from build123d import *

# Parameters (mm, degrees)
F2_DEPTH          = 3
F6_DEPTH          = 1.5
F9_DEPTH          = 26.2
F9_DEPTH_BACK     = 25
F10_R             = 1.5
F11_DEPTH         = 20
F13_R             = 2.25
F14_DEPTH         = 2
F14_COPIES2_COUNT = 2
F14_COPIES2_PITCH = 38.242646
F15_W             = 29
F15_H             = 11
F16_DEPTH         = 0.75


# Not quite as in the source:
# - a pattern or mirror of a feature is missing from the dataset's text; its kind, count and spacing are read off the source's solid


with BuildPart() as f2:
    # F1 (on offset) → F2 (new body)
    with BuildSketch(Plane.XY.offset(3.5)):
        Polygon((-11.75, -15.25), (-11.75, -2.5), (-11.75, 2.5), (-11.75, 15.25), (-16.75, 15.25), (-16.75, 0), (-16.75, -15.25), align=None)
        Polygon((0, -2.5), (11.75, -2.5), (11.75, 2.5), (0, 2.5), (-11.75, 2.5), (-11.75, -2.5), align=None)
        Polygon((16.75, -15.25), (16.75, 0), (16.75, 15.25), (11.75, 15.25), (11.75, 2.5), (11.75, -2.5), (11.75, -15.25), align=None)
    extrude(amount=F2_DEPTH)

    # F5 (on plane+point) → F6 (join, symmetric)
    with BuildSketch(Plane.YZ.offset(14.25)):
        Polygon((10.057664814, 6.5), (13.25, 6.5), (1.5, 38.8), (0, 38.8), (-1.5, 38.8), (-13.25, 6.5), (-10.057664814, 6.5), (-1.5, 30.0244743399), (0, 30.0244743399), (1.5, 30.0244743399), align=None)
    f6 = extrude(amount=F6_DEPTH, both=True)

    # F6_copies: F6 across plane
    add(f6.mirror(Plane(origin=(0, 0, 0), x_dir=(0, 0, -1), z_dir=(-1, 0, 0))))

    # F8 (on face) → F9 (join, two sides)
    with BuildSketch(Plane.XY.offset(38.8)) as f9_sk:
        with BuildLine():
            ThreePointArc((14.25, -1.5), (15.3106601718, -1.0606601718), (15.75, 0))
            ThreePointArc((15.75, 0), (15.3106601718, 1.0606601718), (14.25, 1.5))
            ThreePointArc((14.25, 1.5), (13.1893398223, 1.0606601659), (12.75, -1.67e-08))
            ThreePointArc((12.75, -1.67e-08), (13.1893398341, -1.0606601777), (14.25, -1.5))
        make_face()
    f9 = extrude(amount=F9_DEPTH) + extrude(f9_sk.sketch, amount=-F9_DEPTH_BACK)

    # F9_copies: F9 across plane
    add(f9.mirror(Plane(origin=(0, 0, 0), x_dir=(0, 0, -1), z_dir=(-1, 0, 0))))

    # F10 (on Right) → F11 (join, symmetric)
    with BuildSketch(Plane.YZ):
        with Locations((0, 65)):
            Circle(F10_R)
    extrude(amount=F11_DEPTH, both=True)

    # F13 (on offset) → F14 (join)
    with BuildSketch(Plane.XZ.offset(13.75)):
        with Locations((14.25, 2.25)):
            Circle(F13_R)
    f14 = extrude(amount=-F14_DEPTH)

    # F14_copies: F14 across plane
    add(f14.mirror(Plane.ZX))

    # F14_copies1: F14 across plane
    add(f14.mirror(Plane(origin=(0, 0, 0), x_dir=(0, 0, -1), z_dir=(-1, 0, 0))))

    # F14_copies2: F14 ×2
    with Locations(*[Vector(-0.7452413135, 0.6667948595, 0) * (i * F14_COPIES2_PITCH) for i in range(1, F14_COPIES2_COUNT)]):
        add(f14)

    # F15 (on Front) → F16 (join, symmetric)
    with BuildSketch(Plane.XZ):
        with Locations((0, 71.5)):
            Rectangle(F15_W, F15_H)
    extrude(amount=F16_DEPTH, both=True)


solid = f2.part
Design review of the part built by this model. Coordinates are the model's own, in mm. A direction names the side the tool comes from. Round coordinates to 2 decimals unless told otherwise and drop trailing zeros. Write each loop counter-clockwise with the first axis right and the second up, starting at its lowest first coordinate (ties: lowest second). Pieces come first, ordered by that corner, then holes.
Item 1: Consider section C-C on z = 59.5. Give the boundary of the cut face in (x, y).
Item 2: Consider section A-A on x = -1. Give the boundary of the cut face in (y, z).
Item 3: For faces 1 (the flat face through (11.75, 9, 5)), 2 (the flat face through (15.4, 1.2, 38.8)), 3 (the flat face through (-11.75, -9, 5)), list the 3-axis set-ups (+Z, -Z, +X, -X, +Y, -Y) from which the entire face can be reached by the end or side of a thin tool; tool diameter is ignored.
Item 4: Consider section B-B on z = 2.25. Give the boundary of the cut face in (x, y).
Item 5: Draft analysis for pull direction Z (two halves, no side actions). For faces 4 (the flat face through (14.27, 7.46, 22.42)), 5 (the flat face through (-14.5, 0, 72)), 6 (the flat face through (13.1, 1.2, 30.024)), state which applies: released by +Z, released by -Z, zero draft, split by the parting line, or undercut.
Item 6: For pin 1 Ø5 at (y, z) = (-10, 12.5) entering from -X; pin 2 Ø4 at (x, y) = (10, 6) entering from -Z; pin 3 Ø1.2 at (y, z) = (0, 70) entering from -X; pin 4 Ø4 at (x, z) = (8, 9) entering from +Y, all flat-tipped, find the tip position at first contact; note any pin that passes through.
Item 7: Wall thickness on L1, parallel to Z at x = 6, y = -2; L2, parallel to Y at x = 15, z = 15; L3, parallel to Y at x = 7, z = 72: over which ranges is each line inside the solid? List them lowest first.
Item 8: Consider section D-D on y = 5. Give the boundary of the cut face in (x, z).
Check values:
1. outline: circle Ø3 at (-14.25, 0); circle Ø3 at (14.25, 0)
2. outline: (-2.5, 3.5) - (2.5, 3.5) - (2.5, 6.5) - (-2.5, 6.5) - close; (-0.75, 66.3) arc R1.5 ccw (long way) to (0.75, 66.3) - (0.75, 77) - (-0.75, 77) - close
3. face 1: +Z, -Z, +Y
3. face 2: +X, +Y
3. face 3: +Z, -Z, -Y
4. outline: (-16.5, -13.75) - (-12, -13.75) - (-12, -11.75) - (-16.5, -11.75) - close; (-16.5, 11.75) - (-12, 11.75) - (-12, 13.75) - (-16.5, 13.75) - close; (12, -13.75) - (16.5, -13.75) - (16.5, -11.75) - (12, -11.75) - close; (12, 11.75) - (16.5, 11.75) - (16.5, 13.75) - (12, 13.75) - close
5. face 4: released by +Z
5. face 5: zero draft
5. face 6: undercut
6. pin 1: stops at x = -15.75
6. pin 2: stops at z = 3.5
6. pin 3: stops at x = -14.5
6. pin 4: passes through
7. L1: z = 3.5 to 6.5
7. L2: y = -10.16 to -6.97, -1.3 to 1.3, 6.97 to 10.16
7. L3: y = -0.75 to 0.75
8. outline: (-16.75, 3.5) - (-11.75, 3.5) - (-11.75, 6.5) - (-16.75, 6.5) - close; (-15.75, 20.4) - (-12.75, 20.4) - (-12.75, 29.18) - (-15.75, 29.18) - close; (11.75, 3.5) - (16.75, 3.5) - (16.75, 6.5) - (11.75, 6.5) - close; (12.75, 20.4) - (15.75, 20.4) - (15.75, 29.18) - (12.75, 29.18) - close
